The listing builds one solid part. Answer for the finished solid, in the listing's coordinates (mm). A direction names the side the tool comes from. Give positions to 0.01 mm unless a question says otherwise; leave off trailing zeros. Order: outer loops, then holes, each group sorted by start corner. A loop starts at its lowest first (then second) coordinate and runs counter-clockwise, first axis right, second up. Notation, with made-up numbers: (-30.5, 39) - (-23.5, 39) arc R30 cw to (-23.5, 73) - close; hole circle Ø3 at (-22.75, 35.5). An arc over 180 degrees is marked (long way). Answer in a Markdown table with one row per item.
Autodesk Inventor part; units mm, degrees
ref_plane "YZ Plane" through (0, 0, 0) normal (1, 0, 0) x (0, 1, 0)
ref_plane "XZ Plane" through (0, 0, 0) normal (0, 1, 0) x (-1, 0, 0)
ref_plane "XY Plane" through (0, 0, 0) normal (0, 0, 1) x (1, 0, 0)
sketch "Sketch1" plane through (0, 0, 0) normal (0, 0, 1) x (1, 0, 0)
  line L0 (0, 0) -> (-53, 0)
  line L1 (-53, 0) -> (-53, 33.25) construction
  line L2 (-53, 33.25) -> (0, 33.25)
  line L3 (0, 33.25) -> (0, 0)
  line L4 (-51, 33.25) -> (-51, 0)
  line L5 (0, 0) -> (-51, 0)
  line L6 (-51, 0) -> (-51, -4)
  line L7 (-51, -4) -> (0, -4)
  line L8 (0, -4) -> (0, 0)
  circle A0 centre (-51, 54.6729) radius 54.6729
  line L9 (-26.7487, 5.6729) -> (-2, 30.4216)
  line L10 (-2, 30.4216) -> (-4.8284, 33.25)
  line L11 (-4.8284, 33.25) -> (-29.5772, 8.5013)
  line L12 (-29.5772, 8.5013) -> (-26.7487, 5.6729) construction
  circle A1 centre (-51, 54.6729) radius 47.7965
  line L13 (-29.5772, 8.5013) -> (-31.924, 10.8481)
  circle A2 centre (-51, 54.6729) radius 43.7965
  line L14 (-31.924, 10.8481) -> (-34.9853, 13.9094)
  line L15 (-51, 33.25) -> (0, 33.25)
  line L16 (0, 33.25) -> (0, 37.25)
  line L17 (0, 37.25) -> (-51, 37.25)
  line L18 (-51, 37.25) -> (-51, 33.25)
  line L19 (-4.8284, 33.25) -> (-8.8284, 37.25)
  point P0 (-51, 10.8764)
  point P1 (-51, 6.8764)
  point P2 (-8.2734, 33.25)
  point P3 (-6.4922, 37.25)
  point P4 (-7.1753, 35.5969)
  point P5 (-0.699, 33.25)
  point P6 (0, 34.972)
  dimension "d22" = 95.5929
  dimension "d23" = 87.5929
  dimension "d0" = 53
  dimension "d5" = 51
  dimension "d13" = 4
  dimension "d18" = 35
  dimension "d19" = 4
  dimension "d20" = 2
  dimension "d21" = 45
  dimension "d24" = 4
extrude "Extrusion1" add sketch "Sketch1" along normal blind 44 contours L8 L7 L6 L0 | L0 A0 L2 L3 | L2 A0 L16 | L4 A2 L14 A1 | A0 L10 L2 | L2 L19 A1 L17 L16 A0
extrude "Extrusion2" add sketch "Sketch1" along normal blind 5 contours L8 L7 L6 L0 | L0 A0 L2 L3 | L4 A1 L13 L11 L10 L9 A0 | L4 A2 L14 A1 | L9 A0 | A0 L10 L2 | A1 L11 L13 | L11 A1 L2 | L2 A1 L19
extrude "Extrusion3" add sketch "Sketch1" against normal blind 5 from surface at 44 contours L0 A0 L2 L3 | L4 A1 L13 L11 L10 L9 A0 | L4 A2 L14 A1 | L9 A0 | A0 L10 L2 | L2 L19 A1 L17 L16 A0 | A1 L11 L13 | L11 A1 L2 | L2 A1 L19
sketch "Sketch3" plane through (0, -4, 0) normal (1, 0, 0) x (0, 0, -1)
  line L0 (0, 0) -> (0, 41.25) construction
  line L1 (0, 41.25) -> (-44, 41.25) construction
  line L2 (-44, 0) -> (-44, 41.25) construction
  line L3 (0, 0) -> (-44, 0) construction
  line L4 (-26, 0) -> (-18, 0)
  line L5 (-18, 0) -> (-18, -8)
  line L6 (-18, -8) -> (-26, -8)
  line L7 (-26, -8) -> (-26, 0)
  line L8 (-26, 49.25) -> (-18, 49.25)
  line L9 (-18, 49.25) -> (-18, 41.25)
  line L10 (-18, 41.25) -> (-26, 41.25)
  line L11 (-26, 41.25) -> (-26, 49.25)
  line L12 (-26, 0) -> (-18, -8) construction
  line L13 (-26, 49.25) -> (-18, 41.25) construction
  point P0 (0, 4)
  point P1 (-22, 0)
  point P2 (-22, 41.25)
  point P3 (-22, -4)
  point P4 (-22, 45.25)
  dimension "d33" = 8
  dimension "d34" = 8
  dimension "d35" = 8
  dimension "d36" = 8
extrude "Extrusion5" add sketch "Sketch3" against normal blind 4
sketch "Sketch2" plane through (-51, -4, 0) normal (0, -1, 0) x (1, 0, 0)
  line L0 (30, 26) -> (0, 26)
  line L1 (0, 26) -> (0, 18)
  line L2 (0, 18) -> (30, 18)
  line L3 (30, 18) -> (30, 26)
  line L4 (0, 0) -> (0, 44) construction
  point P0 (51, 0)
  point P1 (0, 22)
  dimension "d29" = 30
  dimension "d30" = 8
extrude "Extrusion4" cut sketch "Sketch2" against normal up to surface
fillet "Fillet2" [suppressed]
chamfer "Chamfer2" [suppressed]
properties part number "Piece-Catch"
Item 1: Which of the six approach directions +Z, -Z, +X, -X, +Y, -Y give full straight-line access (tool end or side, diameter ignored) to faces 1 (the face through (-2, 41, 18)), 2 (the face through (-4.55, 32.97, 21.76)), 3 (the face through (-2, -8, 26)), 4 (the face through (-6.72, 36.68, 23.53)), 5 (the face through (-2, 41, 26))?
Answer block:
| item | result |
|---|---|
| face 1 | -Z, +X, -X, +Y |
| face 2 | -X |
| face 3 | +Z, +X, -X, -Y |
| face 4 | +Z, -Z, +Y |
| face 5 | +Z, +X, -X, +Y |
Item 2: Find section C-C on x = -27.5. Write down the section's boundary in (y, z).
Answer block:
| item | result |
|---|---|
| outline | (-4, 0) - (13.05, 0) - (13.05, 5) - (5.31, 5) - (5.31, 18) - (-4, 18) - close; (-4, 26) - (5.31, 26) - (5.31, 39) - (13.05, 39) - (13.05, 44) - (-4, 44) - close |
Item 3: Find section D-D on y = 12. Write down the section's boundary in (x, z).
Answer block:
| item | result |
|---|---|
| outline | (-41.14, 0) - (-33.08, 0) - (-33.08, 44) - (-41.14, 44) - close; (-29.47, 0) - (0, 0) - (0, 44) - (-29.47, 44) - (-29.47, 39) - (-16.82, 39) - (-16.82, 5) - (-29.47, 5) - close |
Item 4: Each of these flat-tipped pins is pushed along its axis until it touches: P1, Ø4, axis at y = -9.5, z = 22, coming from the -X side; P2, Ø3, axis at x = -2, y = 43, coming from the +Z side; P3, Ø12, axis at x = -15.5, z = 29.5, coming from the -Y side. Where does it stop, or does it pass through?
Answer block:
| item | result |
|---|---|
| P1 | x = -4 |
| P2 | z = 26 |
| P3 | y = -4 |
Item 5: Find section A-A on z = 20.5. Write down the section's boundary in (x, y).
Answer block:
| item | result |
|---|---|
| outline | (-51, 6.88) arc R47.8 ccw to (-31.92, 10.85) - (-34.99, 13.91) arc R43.8 cw to (-51, 10.88) - close; (-21, -4) - (-4, -4) - (-4, -12) - (0, -12) - (0, 45.25) - (-4, 45.25) - (-4, 37.25) - (-6.49, 37.25) arc R47.8 cw to (-7.18, 35.6) - (-2, 30.42) arc R54.67 cw to (-21, 8.97) - close |
Item 6: Determine the mould class of faces 6 (the face through (-25, 13, 39)), 7 (the face through (-20, 8, 44)), 8 (the face through (-4, 41, 22)), 9 (the face through (0, 16, 22)) for opening direction X: pulls with the +X half, pulls with the -X half, needs draft (parallel to the pull), parting line crosses it, or undercut.
Answer block:
| item | result |
|---|---|
| face 6 | undercut |
| face 7 | needs draft |
| face 8 | pulls with the -X half |
| face 9 | pulls with the +X half |
Item 7: Find section B-B on y = -3. Write down the section's boundary in (x, z).
Answer block:
| item | result |
|---|---|
| outline | (-51, 0) - (0, 0) - (0, 44) - (-51, 44) - (-51, 26) - (-21, 26) - (-21, 18) - (-51, 18) - close |
Item 8: Consider line 1 (Z direction, x = -15, y = 18); line 2 (Z direction, x = -35.5, y = 1); line 3 (X direction, y = 10.5, z = 32). Determine where each line is inside the solid, lowest interval first.
Answer block:
| item | result |
|---|---|
| line 1 | 0 to 5, 39 to 44 |
| line 2 | 0 to 18, 26 to 44 |
| line 3 | -51 to -32.74, -18.78 to 0 |
